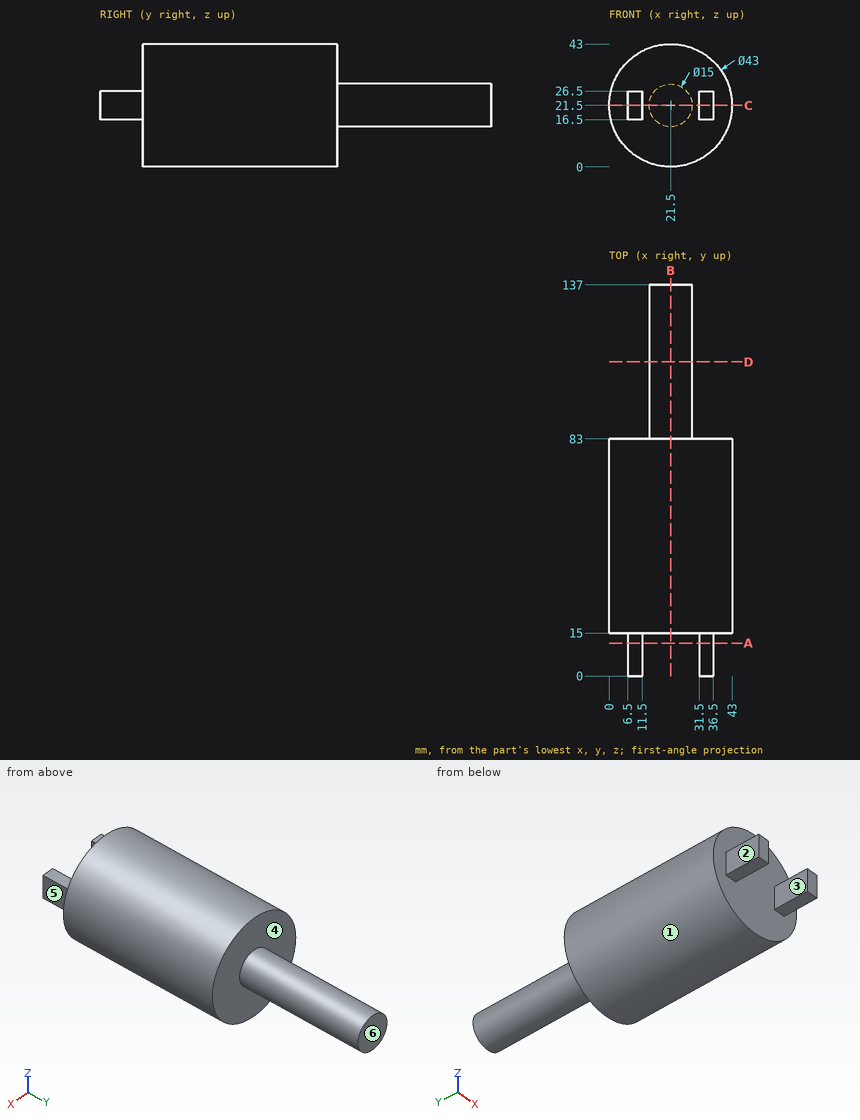
Could you check a few things on this drawing? It's one solid part, dimensions in mm from its lowest x, y, z. A direction names the side the tool comes from. Give positions to 0.01 mm unless a question says otherwise; leave off trailing zeros. Order: outer loops, then holes, each group sorted by start corner. A loop starts at its lowest first (then second) coordinate and runs counter-clockwise, first axis right, second up. Notation, with made-up numbers: (33.5, 73.5) - (85.5, 73.5) arc R19 cw to (85.5, 78.5) - close; hole circle Ø6 at (86, -10). An arc over 180 degrees is marked (long way). One line per item, written item: value. Start each with the question number.
1. Imagine slicing it at C-C on z = 21.5. List the corners of the cut face in (x, y) for me, plus the area to 3 significant figures.
2. For P1, Ø2.5, axis at x = 34, y = 4.5, coming from the -Z side; P2, Ø10, axis at x = 35, y = 14, coming from the -Z side; P3, Ø3, axis at x = 16.5, y = 53.5, coming from the +Z side; P4, Ø10, axis at x = 38, z = 15, coming from the -Y side, each with a flat end and sliding along its axis, tell me the tip position at first contact or that it passes through.
3. If I drill on probe 1 along Y at (x, z) = (39, 15); probe 2 along Z at (x, y) = (22, 64.5); probe 3 along Y at (x, z) = (19.5, 26.5), over which ranges is the centre line in solid material (lowest first)?
4. For the marked faces 4, 5 and 6, which set-ups out of +Z, -Z, +X, -X, +Y, -Y let a thin tool reach every point of the face, with its end or its side?
5. Imagine slicing it at D-D on y = 110. List the corners of the cut face in (x, z) for me, plus the area to 3 significant figures.
6. Imagine slicing it at B-B on x = 21.5. List the corners of the cut face in (y, z) for me, plus the area to 3 significant figures.
7. Imagine slicing it at A-A on y = 11.5. List the corners of the cut face in (x, z) for me, plus the area to 3 significant figures.
8. Thinking about a two-plate mould opening in X: for the marked faces 1, 2 and 3, which applies, +X half, -X half, draft (parallel to the pull), parting line (faces both ways), or undercut?
Values:
1. outline: (0, 15) - (6.5, 15) - (6.5, 0) - (11.5, 0) - (11.5, 15) - (31.5, 15) - (31.5, 0) - (36.5, 0) - (36.5, 15) - (43, 15) - (43, 83) - (29, 83) - (29, 137) - (14, 137) - (14, 83) - (0, 83) - close
1. area: 3,880 mm²
2. P1: z = 16.5
2. P2: z = 1.8
2. P3: z = 42.71
2. P4: y = 0
3. probe 1: 15 to 83
3. probe 2: 0.01 to 42.99
3. probe 3: 15 to 137
4. face 4: +Y
4. face 5: +Z, -Z, +X, -Y
4. face 6: +Z, -Z, +X, -X, +Y
5. outline: circle Ø15 at (21.5, 21.5)
5. area: 177 mm²
6. outline: (15, 0) - (83, 0) - (83, 14) - (137, 14) - (137, 29) - (83, 29) - (83, 43) - (15, 43) - close
6. area: 3,730 mm²
7. outline: (6.5, 16.5) - (11.5, 16.5) - (11.5, 26.5) - (6.5, 26.5) - close; (31.5, 16.5) - (36.5, 16.5) - (36.5, 26.5) - (31.5, 26.5) - close
7. area: 100 mm²
8. face 1: parting line
8. face 2: -X half
8. face 3: undercut
